Geometry check sheet. Reference: the model listing, model coordinates, mm. A direction names the side the tool comes from. Coordinates: 2 decimals unless noted, no trailing zeros. Loops run counter-clockwise (first coordinate to the right, second up) from the corner with the lowest first, then second, coordinate; pieces in that order, holes last. Notation, with made-up numbers: M -24.5,7.25 L -19.5,7.25 A11 ccw -19.5,26.25 Z; hole C 19,37 d2. An arc over 180 degrees is marked long. Use CSV: the item, a comma, the result in double quotes.
```python
from build123d import *

# Parameters (mm, degrees)
F1_DEPTH = 16.66875
F2_R     = 3.571875
F3_DEPTH = 13.833281
F4_R     = 3.175
F4_R_2   = 2.440092
F5_DEPTH = 12.7
F6_R     = 18.25625
F7_DEPTH = 3.81
F8_R     = 1.905
F9_DEPTH = 29.5285


with BuildPart() as f1:
    # F0 (on Front) → F1 (new body, symmetric)
    with BuildSketch(Plane.XZ):
        Polygon((-43.65625, 13.832281), (-43.65625, 0), (43.65625, 0), (43.65625, 13.832281), (24.60625, 13.832281), (24.60625, 50.8), (0, 50.8), (-24.60625, 50.8), (-24.60625, 13.832281), align=None)
    extrude(amount=F1_DEPTH, both=True)

    # F2 (on face) → F3 (cut, through all)
    with BuildSketch(Plane.XY.offset(13.832281)):
        with Locations((-34.13125, 0)):
            Circle(F2_R)
        with Locations((34.13125, 0)):
            Circle(F2_R)
    extrude(amount=-F3_DEPTH, mode=Mode.SUBTRACT)

    # F4 (on face) → F5 (cut)
    with BuildSketch(Plane.XY.offset(50.8)):
        with Locations((15.08125, 0)):
            Circle(F4_R)
        with Locations((-15.197981, 0)):
            Circle(F4_R_2)
    extrude(amount=-F5_DEPTH, mode=Mode.SUBTRACT)

    # F6 (on face) → F7 (cut)
    with BuildSketch(Plane.XZ.offset(16.66875)):
        with Locations((0, 31.75)):
            Circle(F6_R)
    extrude(amount=-F7_DEPTH, mode=Mode.SUBTRACT)

    # F8 (on face) → F9 (cut, through all)
    with BuildSketch(Plane.XZ.offset(12.85875)):
        with Locations((-8.019643, 37.987862)):
            Circle(F8_R)
        with Locations((-0.123209, 41.909253)):
            Circle(F8_R)
        with Locations((7.866004, 38.180519)):
            Circle(F8_R)
        with Locations((9.931956, 29.609473)):
            Circle(F8_R)
        with Locations((4.518942, 22.650288)):
            Circle(F8_R)
        with Locations((-4.296927, 22.543371)):
            Circle(F8_R)
        with Locations((-9.877123, 29.369234)):
            Circle(F8_R)
    extrude(amount=-F9_DEPTH, mode=Mode.SUBTRACT)


solid = f1.part
```
1. Section check A-A, the plane x = 0. Record the cut outline in (y, z).
The answers:
outline,"M -16.67,0 L 16.67,0 L 16.67,40.01 L -12.86,40.01 L -12.86,13.49 L -16.67,13.49 Z; M -16.67,50.01 L -12.86,50.01 L -12.86,43.81 L 16.67,43.81 L 16.67,50.8 L -16.67,50.8 Z"
2. Section check C-C, the plane z = 5. Record the cut outline in (x, y), plus the area to 3 significant figures.
The answers:
outline,"M -43.66,-16.67 L 43.66,-16.67 L 43.66,16.67 L -43.66,16.67 Z; hole C -34.13,0 d7.14; hole C 34.13,0 d7.14"
area,"2,830 mm^2"
3. Set-up check for faces 5 (the flat face through (0, -12.859, 32)), 6 (the flat face through (-34, -4, 13.832)), 7 (the flat face through (43.656, 0, 7)), 8 (the flat face through (34, -4, 13.832)), 9 (the cylindrical face through (-17.636, 0.107, 44.539)): record each of +Z, -Z, +X, -X, +Y, -Y from which the full face is reachable in a straight line by a thin tool's end or side.
The answers:
face 5,"-Y"
face 6,"+Z, -X, +Y, -Y"
face 7,"+Z, -Z, +X, +Y, -Y"
face 8,"+Z, +X, +Y, -Y"
face 9,"+Z"
4. Gauge pin test, flat ends, axial feed: P1, Ø6, axis at x = 4.52, z = 22.65, coming from the -Y side; P2, Ø4, axis at x = -15.5, y = 0, coming from the +Z side; P3, Ø11.5, axis at x = -34.13, y = 0, coming from the +Z side; P4, Ø3, axis at x = 16.5, y = -9, coming from the -Z side. Record the tip position at first contact, or that the pin passes through.
The answers:
P1,"y = -12.86"
P2,"z = 38.1"
P3,"z = 13.83"
P4,"z = 0"
5. Section check D-D, the plane y = -7. Record the cut outline in (x, z) (3 decimals), plus the area to 3 significant figures.
The answers:
outline,"M -43.656,0 L 43.656,0 L 43.656,13.832 L 24.606,13.832 L 24.606,50.8 L -24.606,50.8 L -24.606,13.832 L -43.656,13.832 Z; hole C -9.877,29.369 d3.81; hole C -8.02,37.988 d3.81; hole C -4.297,22.543 d3.81; hole C -0.123,41.909 d3.81; hole C 4.519,22.65 d3.81; hole C 7.866,38.181 d3.81; hole C 9.932,29.609 d3.81"
area,"2,950 mm^2"
6. Section check B-B, the plane y = 0. Count the separate pieces of the cut face and the enclosed holes in it, plus the area to 3 significant figures.
The answers:
separate pieces,"3"
enclosed holes,"7"
area,"2,610 mm^2"
7. Thickness scan on line 1 (Y direction, x = -34, z = 10.5); line 2 (X direction, y = 12, z = 39); line 3 (X direction, y = 10.5, z = 24). Record the ranges inside material, lowest first. Write a range as [from, to].
The answers:
line 1,"[-16.67, -3.57], [3.57, 16.67]"
line 2,"[-24.61, -9.63], [-6.41, 6.15], [9.59, 24.61]"
line 3,"[-24.61, -5.52], [-3.07, 3.17], [5.86, 24.61]"
8. Release check for a two-part mould opening along Y. For faces 1 (the cylindrical face through (-8.06, 1.7, 29.94)), 2 (the cylindrical face through (12.56, -1.93, 44.54)), 3 (the cylindrical face through (-30.724, 1.073, 7.013)), 4 (the flat face through (-1, 16.669, 20)) record: +Y half, -Y half, draft (parallel to the pull), parting line (faces both ways), or undercut.
The answers:
face 1,"draft"
face 2,"undercut"
face 3,"undercut"
face 4,"+Y half"
